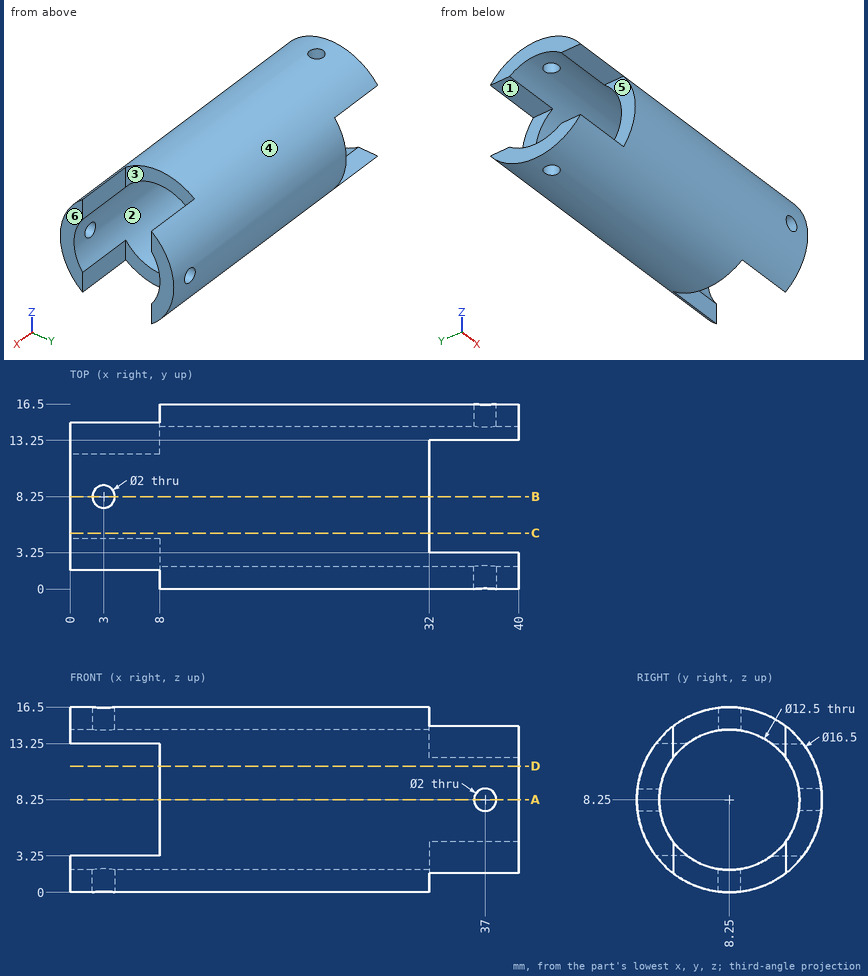
Can you work these out from the drawing? Everything is in mm from the part's minimum corner. A direction names the side the tool comes from. Round coordinates to 2 decimals unless told otherwise and drop trailing zeros. Write each loop counter-clockwise with the first axis right and the second up, starting at its lowest first coordinate (ties: lowest second). Pieces come first, ordered by that corner, then holes.
1. If we mould it in two halves opening along Z, with no side actions, what happens to the marked faces 4, 5 and 6? For each: released by +Z, released by -Z, zero draft, split by the parting line, or undercut.
2. Suppose I cut it at B-B (y = 8.25). List the corners of the cut face in (x, z) for me, and give its area (3 significant figures).
3. Suppose I cut it at D-D (z = 11.25). List the corners of the cut face in (x, y) for me.
4. I need wall thicknesses on L1, parallel to Y at x = 26, z = 3.25; L2, parallel to Z at x = 32.5, y = 13.5. Which ranges of each line are inside material? Lowest first, please.
5. Suppose I cut it at A-A (z = 8.25). List the corners of the cut face in (x, y) for me.
6. Suppose I cut it at C-C (y = 5). List the corners of the cut face in (x, z) for me, and give its area (3 significant figures).
7. For the marked faces 1, 2 and 3, which set-ups out of +Z, -Z, +X, -X, +Y, -Y let a thin tool reach every point of the face, with its end or its side?
8. Will these pins go through, and if not, where does the flat tip stop? pin 1 Ø3 at (x, y) = (31, 2) entering from +Z; pin 2 Ø0.8 at (x, z) = (36, 13.5) entering from +Y; pin 3 Ø1.4 at (x, z) = (38, 3.5) entering from -Y; pin 4 Ø2.5 at (x, y) = (3, 8.25) entering from +Z.
Answer sheet:
1. face 4: split by the parting line
1. face 5: undercut
1. face 6: zero draft
2. outline: (0, 0) - (2, 0) - (2, 2) - (0, 2) - close; (0, 14.5) - (2, 14.5) - (2, 16.5) - (0, 16.5) - close; (4, 0) - (32, 0) - (32, 2) - (4, 2) - close; (4, 14.5) - (32, 14.5) - (32, 16.5) - (4, 16.5) - close
2. area: 120 mm2
3. outline: (8, 0.56) - (40, 0.56) - (40, 2.77) - (8, 2.77) - close; (8, 13.73) - (40, 13.73) - (40, 15.94) - (8, 15.94) - close
4. L1: y = 1.69 to 4.5, 12 to 14.81
4. L2: z = 1.89 to 4.86, 11.64 to 14.61
5. outline: (8, 0) - (36, 0) - (36, 2) - (8, 2) - close; (8, 14.5) - (36, 14.5) - (36, 16.5) - (8, 16.5) - close; (38, 0) - (40, 0) - (40, 2) - (38, 2) - close; (38, 14.5) - (40, 14.5) - (40, 16.5) - (38, 16.5) - close
6. outline: (0, 0.67) - (32, 0.67) - (32, 2.91) - (0, 2.91) - close; (0, 13.59) - (32, 13.59) - (32, 15.83) - (0, 15.83) - close
6. area: 144 mm2
7. face 1: -X, +Y, -Y
7. face 2: +X, -X
7. face 3: +Z, -Z, +X
8. pin 1: stops at z = 15
8. pin 2: stops at y = 14.92
8. pin 3: stops at y = 1.06
8. pin 4: stops at z = 16.5
